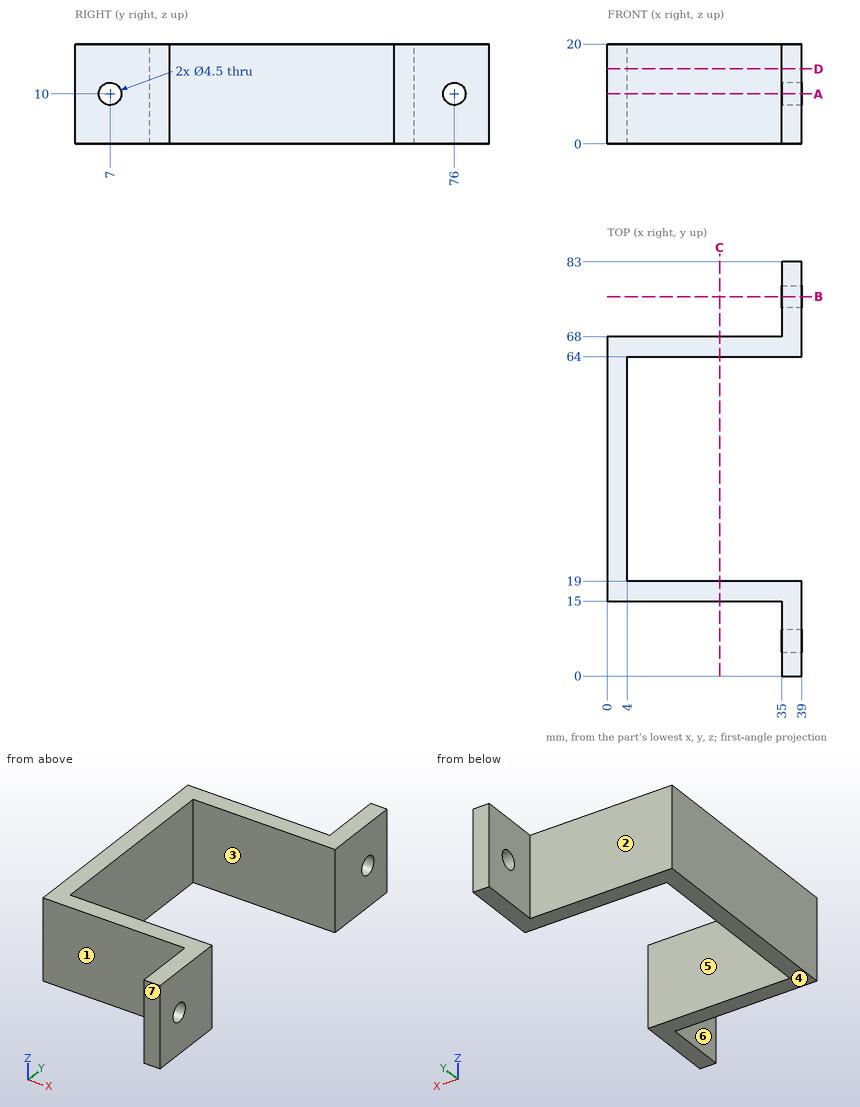
Design review of the part shown in the three views and the two pictorial views. Dimensions are in mm from the part's minimum x, y and z. A direction names the side the tool comes from. Coordinates: 2 decimals unless noted, no trailing zeros. Order: outer loops, then holes, each group sorted by start corner. A loop starts at its lowest first (then second) coordinate and runs counter-clockwise, first axis right, second up. Notation, with made-up numbers: (38.5, 34.25) -> (82.5, 34.25) arc R23 ccw to (82.5, 48.25) -> close; hole circle Ø10 at (72.5, 6). An arc over 180 degrees is marked (long way). Use one line per item in the form item = value. Start each with the question number.
(1) The part is to be moulded in two halves that separate along Y. For the marked faces 5, 6 and 7, say which applies: +Y half, -Y half, draft (parallel to the pull), parting line (faces both ways), or undercut.
(2) For the marked faces 1, 2, 3 and 4, list the 3-axis set-ups (+Z, -Z, +X, -X, +Y, -Y) from which the entire face can be reached by the end or side of a thin tool; tool diameter is ignored.
(3) Insertion check: pin 1 (6 mm diameter, centred on x = 21, z = 13.5, fed in from +Y); pin 2 (4 mm diameter, centred on x = 31, z = 11, fed in from -Y); pin 3 (6 mm diameter, centred on y = 22.5, z = 4.5, fed in from +X); pin 4 (3.5 mm diameter, centred on y = 76, z = 10, fed in from -X). Each pin has a flat end and moves straight along its axis. Give the tip position at first contact, or say it passes through.
(4) Add section D-D on z = 15. State the section outline as (x, y) points, plus the area to 3 significant figures.
(5) Add section B-B on y = 76. State the section outline as (x, z) points, plus the area to 3 significant figures.
(6) Add section C-C on x = 22.5. State the section outline as (y, z) points, plus the area to 3 significant figures.
(7) Add section A-A on z = 10. State the section outline as (x, y) points.
(8) For probe 1 along Y at (x, z) = (32, 14.5); probe 2 along Z at (x, y) = (37, 7); probe 3 along X at (y, z) = (30, 12), list the stretches that pass through material, from the lowest coordinate up.
Answer block:
q1.face_5 = undercut
q1.face_6 = draft
q1.face_7 = -Y half
q2.face_1 = +Z, -Z, -X, -Y
q2.face_2 = +Z, -Z, -X, +Y
q2.face_3 = +Z, -Z, +X
q2.face_4 = -Z, +X, -X, +Y, -Y
q3.pin_1 = 68
q3.pin_2 = 15
q3.pin_3 = 4
q3.pin_4 = through
q4.outline = (0, 15) -> (35, 15) -> (35, 0) -> (39, 0) -> (39, 19) -> (4, 19) -> (4, 64) -> (39, 64) -> (39, 83) -> (35, 83) -> (35, 68) -> (0, 68) -> close
q4.area = 612 mm²
q5.outline = (35, 0) -> (39, 0) -> (39, 7.75) -> (35, 7.75) -> close; (35, 12.25) -> (39, 12.25) -> (39, 20) -> (35, 20) -> close
q5.area = 62.0 mm²
q6.outline = (15, 0) -> (19, 0) -> (19, 20) -> (15, 20) -> close; (64, 0) -> (68, 0) -> (68, 20) -> (64, 20) -> close
q6.area = 160 mm²
q7.outline = (0, 15) -> (35, 15) -> (35, 9.25) -> (39, 9.25) -> (39, 19) -> (4, 19) -> (4, 64) -> (39, 64) -> (39, 73.75) -> (35, 73.75) -> (35, 68) -> (0, 68) -> close; (35, 0) -> (39, 0) -> (39, 4.75) -> (35, 4.75) -> close; (35, 78.25) -> (39, 78.25) -> (39, 83) -> (35, 83) -> close
q8.probe_1 = 15 to 19, 64 to 68
q8.probe_2 = 0 to 7.75, 12.25 to 20
q8.probe_3 = 0 to 4
